```python
from build123d import *

# Parameters (mm, degrees)
SKETCH_R     = 22.5
SKETCH_R_2   = 15
PAD_DEPTH    = 8
SKETCH001_R  = 4
POCKET_DEPTH = 22.501
CHAMFER_SIZE = 1


with BuildPart() as part:
    # Sketch → Pad (new body, symmetric)
    with BuildSketch(Plane.XY):
        Circle(SKETCH_R)
        Circle(SKETCH_R_2, mode=Mode.SUBTRACT)
    extrude(amount=PAD_DEPTH, both=True)

    # Sketch001 → Pocket (cut, through all)
    with BuildSketch(Plane.XZ):
        Circle(SKETCH001_R)
    extrude(amount=-POCKET_DEPTH, mode=Mode.SUBTRACT)

    # Chamfer
    chamfer_edges = [part.edges().sort_by_distance(p)[0] for p in [
        (-15, 0, -8),
        (-22.5, 0, -8),
        (-15, 0, 8),
        (-22.5, 0, 8),
    ]]
    chamfer(chamfer_edges, length=CHAMFER_SIZE)


solid = part.part
```
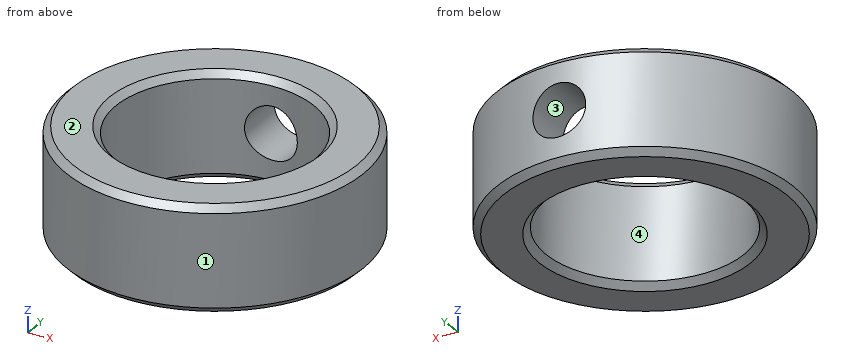
Geometry: final body of the model. Coordinates: model frame, mm. Face numbers are marked on the shaded views. Coordinates: 2 decimals unless noted, no trailing zeros. Loops run counter-clockwise (first coordinate to the right, second up) from the corner with the lowest first, then second, coordinate; pieces in that order, holes last. Notation, with made-up numbers: (-1, -28) -> (50, -28) arc R17 cw to (50, -16) -> close; hole circle Ø10 at (-33, -22). An arc over 180 degrees is marked (long way). Use a Markdown table: item, result. Add a question column.
(1) Section query D-D, the plane z = 0. Return loops of the section in (x, y), plus the area to 3 significant figures.
(2) Mould query, pull axis X, two halves, no side actions, for the marked faces 1, 2, 3 and 4. Classes: pulls with the +X half, pulls with the -X half, needs draft (parallel to the pull), parting line crosses it, or undercut.
(3) Section query C-C, the plane z = -3.25. Return loops of the section in (x, y), plus the area to 4 significant figures.
(4) Line query: line 1 along Z through (x, y) = (0, 17.5); line 2 along X through (y, z) = (0.5, 2.25); line 3 along X through (y, z) = (18.25, 0). Output: solid intervals per line, ascending.
(5) Pin query (flat end, axial travel): pin 1 Ø3 at (y, z) = (-12, -3.5) entering from +X; pin 2 Ø6 at (x, z) = (-2.5, -3.5) entering from -Y; pin 3 Ø5 at (x, z) = (-10, -0.5) entering from -Y; pin 4 Ø12 at (x, y) = (13.5, -17.5) entering from +Z. Return the tip coordinate at first contact, or that it passes through.
(6) Section query A-A, the plane x = 0. Return loops of the section in (y, z).
(7) Section query B-B, the plane y = 0. Return loops of the section in (x, z), plus the area to 3 significant figures.
Answer:
| question | item | result |
|---|---|---|
| 1 | outline | (-4, 14.46) -> (-4, 22.14) arc R22.5 ccw (long way) to (4, 22.14) -> (4, 14.46) arc R15 cw (long way) to start |
| 1 | area | 823 mm^2 |
| 2 | face 1 | parting line crosses it |
| 2 | face 2 | needs draft |
| 2 | face 3 | undercut |
| 2 | face 4 | undercut |
| 3 | outline | (-2.33, 14.82) -> (-2.33, 22.38) arc R22.5 ccw (long way) to (2.33, 22.38) -> (2.33, 14.82) arc R15 cw (long way) to start |
| 3 | area | 848.5 mm^2 |
| 4 | line 1 | z = -8 to -4, 4 to 8 |
| 4 | line 2 | x = -22.49 to -14.99, 14.99 to 22.49 |
| 4 | line 3 | x = -13.16 to -4, 4 to 13.16 |
| 5 | pin 1 | stops at x = 19.9 |
| 5 | pin 2 | stops at y = -22.5 |
| 5 | pin 3 | stops at y = -21.21 |
| 5 | pin 4 | stops at z = 8 |
| 6 | outline | (-22.5, -7) -> (-21.5, -8) -> (-16, -8) -> (-15, -7) -> (-15, 7) -> (-16, 8) -> (-21.5, 8) -> (-22.5, 7) -> close; (15, -7) -> (16, -8) -> (21.5, -8) -> (22.5, -7) -> (22.5, -4) -> (15, -4) -> close; (15, 4) -> (22.5, 4) -> (22.5, 7) -> (21.5, 8) -> (16, 8) -> (15, 7) -> close |
| 7 | outline | (-22.5, -7) -> (-21.5, -8) -> (-16, -8) -> (-15, -7) -> (-15, 7) -> (-16, 8) -> (-21.5, 8) -> (-22.5, 7) -> close; (15, -7) -> (16, -8) -> (21.5, -8) -> (22.5, -7) -> (22.5, 7) -> (21.5, 8) -> (16, 8) -> (15, 7) -> close |
| 7 | area | 236 mm^2 |
